from build123d import *

# Parameters (mm, degrees)
F1_DEPTH = 5
F2_D     = 6.3
F3_SIZE  = 3
F4_W     = 8.1
F4_H     = 6.85
F4_W_2   = 6.85
F4_H_2   = 8.1
F4_W_3   = 27.7
F5_DEPTH = 2
F6_R     = 1.5


with BuildPart() as f1:
    # F0 (on Top) → F1 (new body)
    with BuildSketch(Plane.XY):
        Polygon((-35, 28), (-35, 0), (35, 0), (35, 28), (14, 47), (14, 59), (-14, 59), (-14, 47), align=None)
    extrude(amount=-F1_DEPTH)

    # F2 (through all)
    with Locations(Plane.XY):
        with Locations((20, 14), (-20, 14), (0, 44)):
            Hole(F2_D / 2)

    # F3
    f3_edges = [f1.edges().sort_by_distance(p)[0] for p in [
        (14, 59, -2.5),
        (-14, 59, -2.5),
        (35, 0, -2.5),
        (-35, 0, -2.5),
    ]]
    chamfer(f3_edges, length=F3_SIZE)

    # F4 (on face) → F5 (join)
    with BuildSketch(Plane.XY):
        with Locations((0, 53.575)):
            Rectangle(F4_W, F4_H)
        with Locations((0, 34.425)):
            Rectangle(F4_W, F4_H)
        with Locations((29.575, 14)):
            Rectangle(F4_W_2, F4_H_2)
        with Locations((0, 14)):
            Rectangle(F4_W_3, F4_H_2)
        with Locations((-29.575, 14)):
            Rectangle(F4_W_2, F4_H_2)
    extrude(amount=F5_DEPTH)

    # F6
    f6_edges = [f1.edges().sort_by_distance(p)[0] for p in [
        (-26.15, 9.95, 1),
        (-33, 9.95, 1),
        (-33, 18.05, 1),
        (-26.15, 18.05, 1),
        (-13.85, 9.95, 1),
        (-13.85, 18.05, 1),
        (13.85, 9.95, 1),
        (13.85, 18.05, 1),
        (33, 18.05, 1),
        (33, 9.95, 1),
        (26.15, 9.95, 1),
        (26.15, 18.05, 1),
        (4.05, 31, 1),
        (-4.05, 31, 1),
        (4.05, 37.85, 1),
        (-4.05, 37.85, 1),
        (4.05, 57, 1),
        (4.05, 50.15, 1),
        (-4.05, 57, 1),
        (-4.05, 50.15, 1),
    ]]
    fillet(f6_edges, radius=F6_R)


solid = f1.part
Input: part model. Units: mm. Frame: model coordinates. A direction names the side the tool comes from. Round coordinates to 2 decimals unless told otherwise and drop trailing zeros. Loops run counter-clockwise (first coordinate to the right, second up) from the corner with the lowest first, then second, coordinate; pieces in that order, holes last. Notation, with made-up numbers: M 52,13 L 77,13 A12 ccw 77,24 Z; hole C 59,-19.75 d4. An arc over 180 degrees is marked long. Answer as CSV lines item,"result". Start each with the question number.
(1) Section D-D, the plane x = 0. Output: boundary loops of the cut face in (y, z), plus the area to 3 significant figures.
(2) Draft query along Y for faces 1 (the cylindrical face through (32.55, 10.38, 1.01)), 2 (the cylindrical face through (3.6, 31.43, 1.01)), 3 (the cylindrical face through (-3.6, 56.57, 1.01)). Return one class per face: released by +Y, released by -Y, zero draft, split by the parting line, or undercut.
(3) First-contact query: pin 1 (1 mm diameter, centred on x = -1, z = 1, fed in from +Y); pin 2 (1 mm diameter, centred on y = 34, z = 1.5, fed in from +X); pin 3 (8 mm diameter, centred on x = 11, y = 36.5, fed in from +Z); pin 4 (7 mm diameter, centred on x = 0, y = 44, fed in from -Z). Flat tips, straight axial feed; report the tip coordinate or a pass-through.
(4) Section B-B, the plane x = 8. Output: boundary loops of the cut face in (y, z), plus the area to 3 significant figures.
(5) Line query: line 1 (Y direction, x = 0, z = -2.35); line 2 (X direction, y = 14.5, z = -3.75); line 3 (Y direction, x = -28, z = 0.25). Output: solid intervals per line, ascending. Write a range as [from, to].
(6) Section A-A, the plane y = 14. Output: boundary loops of the cut face in (x, z), plus the area to 3 significant figures.
(7) Section C-C, the plane z = -3.75. Output: boundary loops of the cut face in (x, y), plus the area to 3 significant figures.
(8) Reachability of faces 4 (the cylindrical face through (-26.58, 17.6, 1.01)), 5 (the cylindrical face through (-32.55, 17.62, 1.01)), 6 (the flat face through (0, 9.95, 1)) from +Z, -Z, +X, -X, +Y, -Y: full face, straight path, thin tool, end or side. Return the list, or none.
Values found:
1,outline,"M 0,-5 L 40.85,-5 L 40.85,0 L 37.85,0 L 37.85,2 L 31,2 L 31,0 L 18.05,0 L 18.05,2 L 9.95,2 L 9.95,0 L 0,0 Z; M 47.15,-5 L 59,-5 L 59,0 L 57,0 L 57,2 L 50.15,2 L 50.15,0 L 47.15,0 Z"
1,area,"307 mm²"
2,face 1,"released by -Y"
2,face 2,"undercut"
2,face 3,"released by +Y"
3,pin 1,"stops at y = 57"
3,pin 2,"stops at x = 4.05"
3,pin 3,"stops at z = 0"
3,pin 4,"stops at z = -5"
4,outline,"M 0,-5 L 59,-5 L 59,0 L 18.05,0 L 18.05,2 L 9.95,2 L 9.95,0 L 0,0 Z"
4,area,"311 mm²"
5,line 1,"y = [0, 40.85], [47.15, 59]"
5,line 2,"x = [-35, -23.11], [-16.89, 16.89], [23.11, 35]"
5,line 3,"y = [9.95, 18.05]"
6,outline,"M -35,-5 L -23.15,-5 L -23.15,0 L -26.15,0 L -26.15,2 L -33,2 L -33,0 L -35,0 Z; M -16.85,-5 L 16.85,-5 L 16.85,0 L 13.85,0 L 13.85,2 L -13.85,2 L -13.85,0 L -16.85,0 Z; M 23.15,-5 L 35,-5 L 35,0 L 33,0 L 33,2 L 26.15,2 L 26.15,0 L 23.15,0 Z"
6,area,"370 mm²"
7,outline,"M -35,3 L -32,0 L 32,0 L 35,3 L 35,28 L 14,47 L 14,56 L 11,59 L -11,59 L -14,56 L -14,47 L -35,28 Z; hole C -20,14 d6.3; hole C 0,44 d6.3; hole C 20,14 d6.3"
7,area,"3,120 mm²"
8,face 4,"+Z, +Y"
8,face 5,"+Z, -X, +Y"
8,face 6,"+Z, +X, -X, -Y"
